```python
from build123d import *

# Parameters (mm, degrees)
SKETCH1_W           = 200
SKETCH1_H           = 180
SKETCH1_R           = 1
SKETCH1_R_2         = 6
SKETCH1_W_2         = 140
SKETCH1_H_2         = 140
BOSS_EXTRUDE4_DEPTH = 3
SKETCH1_3_W         = 204
SKETCH1_3_H         = 184
SKETCH1_3_W_2       = 200
SKETCH1_3_H_2       = 180
BOSS_EXTRUDE5_DEPTH = 10
SKETCH4_R           = 1
CUT_EXTRUDE1_DEPTH  = 2
SKETCH7_R           = 1
CUT_EXTRUDE2_DEPTH  = 2
CUT_EXTRUDE3_START  = -2
SKETCH6_R           = 1
CUT_EXTRUDE3_DEPTH  = 2
CUT_EXTRUDE4_START  = -2
SKETCH5_R           = 1
CUT_EXTRUDE4_DEPTH  = 2


with BuildPart() as part:
    # Sketch1 → Boss-Extrude4 (new body)
    with BuildSketch(Plane(origin=(0, 0, 0), x_dir=(1, 0, 0), z_dir=(0, 1, 0))):
        Rectangle(SKETCH1_W, SKETCH1_H)
        with Locations(Location((85, -20, 0), (0, 0, 270))):
            Circle(SKETCH1_R, mode=Mode.SUBTRACT)
        with Locations(Location((90, 49.146026748, 0), (0, 0, 270))):
            Circle(SKETCH1_R_2, mode=Mode.SUBTRACT)
        with Locations(Location((90, -49.146026748, 0), (0, 0, 270))):
            Circle(SKETCH1_R_2, mode=Mode.SUBTRACT)
        with Locations(Location((90, -80, 0), (0, 0, 270))):
            Circle(SKETCH1_R_2, mode=Mode.SUBTRACT)
        with Locations(Location((-90, -80, 0), (0, 0, 270))):
            Circle(SKETCH1_R_2, mode=Mode.SUBTRACT)
        with Locations(Location((-90, 49.146026748, 0), (0, 0, 270))):
            Circle(SKETCH1_R_2, mode=Mode.SUBTRACT)
        with Locations(Location((-90, 80, 0), (0, 0, 270))):
            Circle(SKETCH1_R_2, mode=Mode.SUBTRACT)
        with Locations(Location((-85, 20, 0), (0, 0, 270))):
            Circle(SKETCH1_R, mode=Mode.SUBTRACT)
        with Locations(Location((5, 80, 0), (0, 0, 270))):
            Circle(SKETCH1_R, mode=Mode.SUBTRACT)
        with Locations(Location((5, -80, 0), (0, 0, 270))):
            Circle(SKETCH1_R, mode=Mode.SUBTRACT)
        with Locations(Location((-90, -49.146026748, 0), (0, 0, 270))):
            Circle(SKETCH1_R_2, mode=Mode.SUBTRACT)
        with Locations(Location((90, 80, 0), (0, 0, 270))):
            Circle(SKETCH1_R_2, mode=Mode.SUBTRACT)
        Rectangle(SKETCH1_W_2, SKETCH1_H_2, mode=Mode.SUBTRACT)
    extrude(amount=BOSS_EXTRUDE4_DEPTH)

    # Sketch1_3 → Boss-Extrude5 (add)
    with BuildSketch(Plane(origin=(0, 0, 0), x_dir=(1, 0, 0), z_dir=(0, 1, 0))):
        Rectangle(SKETCH1_3_W, SKETCH1_3_H)
        Rectangle(SKETCH1_3_W_2, SKETCH1_3_H_2, mode=Mode.SUBTRACT)
    extrude(amount=BOSS_EXTRUDE5_DEPTH)

    # Sketch4 → Cut-Extrude1 (cut)
    with BuildSketch(Plane.ZY.offset(102)):
        with Locations((0, 8)):
            Circle(SKETCH4_R)
    extrude(amount=-CUT_EXTRUDE1_DEPTH, mode=Mode.SUBTRACT)

    # Sketch7 → Cut-Extrude2 (cut)
    with BuildSketch(Plane(origin=(0, 0, -92), x_dir=(-1, 0, 0), z_dir=(0, 0, -1))):
        with Locations((0, 8)):
            Circle(SKETCH7_R)
    extrude(amount=-CUT_EXTRUDE2_DEPTH, mode=Mode.SUBTRACT)

    # Sketch6 → Cut-Extrude3 (cut)
    with BuildSketch(Plane(origin=(102, 0, 0), x_dir=(0, 0, -1), z_dir=(1, 0, 0)).offset(CUT_EXTRUDE3_START)):
        with Locations(Location((0, 8, 0), (0, 0, 180))):
            Circle(SKETCH6_R)
    extrude(amount=CUT_EXTRUDE3_DEPTH, mode=Mode.SUBTRACT)

    # Sketch5 → Cut-Extrude4 (cut)
    with BuildSketch(Plane.XY.offset(92).offset(CUT_EXTRUDE4_START)):
        with Locations(Location((0, 8, 0), (0, 0, 180))):
            Circle(SKETCH5_R)
    extrude(amount=CUT_EXTRUDE4_DEPTH, mode=Mode.SUBTRACT)


solid = part.part
```
Geometry check sheet. Reference: the model listing, model coordinates, mm. A direction names the side the tool comes from. Round coordinates to 2 decimals unless told otherwise and drop trailing zeros. Order: outer loops, then holes, each group sorted by start corner. A loop starts at its lowest first (then second) coordinate and runs counter-clockwise, first axis right, second up. Notation, with made-up numbers: (42, 23) -> (69, 23) arc R14 ccw to (69, 38) -> close; hole circle Ø10 at (84, -9.5). An arc over 180 degrees is marked (long way). Return JSON: item names as keys, results as strings. Group by question number.
Q1. Section check B-B, the plane z = -36.5. Record the boundary of the cut face in (x, y).
Q2. Tool access check on faces 5 (the flat face through (-1, 5, -92)), 6 (the flat face through (-8, 3, 73)). Record the directions out of +Z, -Z, +X, -X, +Y, -Y that give a thin tool (end or side, any length) a straight path to the whole face; none if there is none.
Q3. Section check A-A, the plane y = 5.25. Record the boundary of the cut face in (x, z).
Q4. Material ranges on probe 1 along X at (y, z) = (0.5, -48.5); probe 2 along X at (y, z) = (2, -80); probe 3 along Z at (x, y) = (50, 4.5), recorded low to high. Write a range as from..to.
Q5. Section check C-C, the plane x = -90. Record the boundary of the cut face in (y, z), plus the area to 3 significant figures.
Q6. Gauge pin test, flat ends, axial feed: pin 1 (11 mm diameter, centred on x = 90, z = -80, fed in from +Y); pin 2 (14 mm diameter, centred on x = -90, z = -49.15, fed in from +Y). Record the tip position at first contact, or that the pin passes through.
Q7. Release check for a two-part mould opening along X. For faces 1 (the cylindrical face through (95.06, 1.48, -45.92)), 2 (the flat face through (102, 5, 1)), 3 (the flat face through (-102, 5, 1)), 4 (the flat face through (-8, 0, -75)) record: released by +X, released by -X, zero draft, split by the parting line, or undercut.
Numbers:
{
 "1": {"outline": "(-102, 0) -> (-70, 0) -> (-70, 3) -> (-100, 3) -> (-100, 10) -> (-102, 10) -> close; (70, 0) -> (102, 0) -> (102, 10) -> (100, 10) -> (100, 3) -> (70, 3) -> close"},
 "2": {"face 5": "-Z, +X, -X, +Y, -Y", "face 6": "+Y"},
 "3": {"outline": "(-102, -92) -> (102, -92) -> (102, 92) -> (-102, 92) -> close; hole (-100, -90) -> (100, -90) -> (100, 90) -> (-100, 90) -> close"},
 "4": {"probe 1": "-102..-95.97, -84.03..-70, 70..84.03, 95.97..102", "probe 2": "-102..-96, -84..4, 6..84, 96..102", "probe 3": "-92..-90, 90..92"},
 "5": {"outline": "(0, -92) -> (10, -92) -> (10, -90) -> (3, -90) -> (3, -86) -> (0, -86) -> close; (0, -74) -> (3, -74) -> (3, -55.15) -> (0, -55.15) -> close; (0, -43.15) -> (3, -43.15) -> (3, 43.15) -> (0, 43.15) -> close; (0, 55.15) -> (3, 55.15) -> (3, 74) -> (0, 74) -> close; (0, 86) -> (3, 86) -> (3, 90) -> (10, 90) -> (10, 92) -> (0, 92) -> close", "area": "436 mm^2"},
 "6": {"pin 1": "through", "pin 2": "y = 3"},
 "7": {"face 1": "undercut", "face 2": "released by +X", "face 3": "released by -X", "face 4": "zero draft"}
}
